Check sheet for the modelled part. Datum: model origin and axes. Units: mm. Coordinates: 2 decimals unless noted, no trailing zeros. Write each loop counter-clockwise with the first axis right and the second up, starting at its lowest first coordinate (ties: lowest second). Pieces come first, ordered by that corner, then holes. Notation, with made-up numbers: M 30,-9.75 L 81,-9.75 A12 cw 81,-4.75 Z; hole C -19.5,38.25 d6. An arc over 180 degrees is marked long. Answer as CSV lines item,"result". Start each with the question number.
1) Draft check along X on faces 1 (the cylindrical face through (-40.4, -86.24, 3.94)), 2 (the cylindrical face through (21.758, -75.637, 3.944)), 3 (the cylindrical face through (-1.788, -84.054, 3.944)), 4 (the flat face through (1, -33, 0)). Enter one of: +X half, -X half, draft (parallel to the pull), parting line (faces both ways), or undercut.
2) Material ranges on L1, parallel to X at y = -4.5, z = 4; L2, parallel to Y at x = -27, z = 1.75; L3, parallel to Y at x = -30, z = 6, recorded low to high. Write a range as [from, to].
3) Go/stop test with flat-tipped pins: pin 1 Ø21.5 at (x, y) = (30, -76) entering from -Z; pin 2 Ø4 at (y, z) = (-11.5, 6.5) entering from +X. Record where each tip stops, or that it passes through.
4) Section check C-C (x = -31.5). Record the cut outline in (y, z), and give its area (3 significant figures).
5) Section check B-B (z = 2.5). Record the cut outline in (x, y).
6) Section check A-A (y = -76). Record the cut outline in (x, z), and give its area (3 significant figures).
7) Section check D-D (x = 0). Record the cut outline in (y, z).
from build123d import *

# Parameters (mm, degrees)
SKETCH_R   = 8
SKETCH_R_2 = 8.25
PAD_DEPTH  = 8


with BuildPart() as part:
    # Sketch → Pad (new body)
    with BuildSketch(Plane.XY):
        with BuildLine():
            Line((-43.25, -79.25), (-43.25, -29.25))
            ThreePointArc((-39.101298, -16.231558), (-42.18775, -22.418244), (-43.25, -29.25))
            Line((-39.101298, -16.231558), (-18.351298, 13.018442))
            ThreePointArc((18.351298, 13.018442), (0, 22.5), (-18.351298, 13.018442))
            Line((39.101298, -16.231558), (18.351298, 13.018442))
            ThreePointArc((43.25, -29.25), (42.18775, -22.418244), (39.101298, -16.231558))
            Line((43.25, -79.25), (43.25, -29.25))
            ThreePointArc((33.25, -89.25), (40.321068, -86.321068), (43.25, -79.25))
            Line((-33.25, -89.25), (33.25, -89.25))
            ThreePointArc((-43.25, -79.25), (-40.321068, -86.321068), (-33.25, -89.25))
        make_face()
        Circle(SKETCH_R, mode=Mode.SUBTRACT)
        with Locations((0, -76)):
            Circle(SKETCH_R_2, mode=Mode.SUBTRACT)
        with Locations((30, -76)):
            Circle(SKETCH_R_2, mode=Mode.SUBTRACT)
        with Locations((-30, -76)):
            Circle(SKETCH_R_2, mode=Mode.SUBTRACT)
    extrude(amount=PAD_DEPTH)


solid = part.part
Results found:
1,face 1,"-X half"
1,face 2,"undercut"
1,face 3,"undercut"
1,face 4,"draft"
2,L1,"x = [-30.78, -6.61], [6.61, 30.78]"
2,L2,"y = [-89.25, -83.69], [-68.31, 0.83]"
2,L3,"y = [-89.25, -84.25], [-67.75, -3.4]"
3,pin 1,"stops at z = 0"
3,pin 2,"stops at x = 37.16"
4,outline,"M -89.25,0 L -84.11,0 L -84.11,8 L -89.25,8 Z; M -67.89,0 L -5.52,0 L -5.52,8 L -67.89,8 Z"
4,area,"540 mm2"
5,outline,"M -43.25,-79.25 A10 ccw -33.25,-89.25 L 33.25,-89.25 A10 ccw 43.25,-79.25 L 43.25,-29.25 A22.5 ccw 39.1,-16.23 L 18.35,13.02 A22.5 ccw -18.35,13.02 L -39.1,-16.23 A22.5 ccw -43.25,-29.25 Z; hole C -30,-76 d16.5; hole C 0,-76 d16.5; hole C 0,0 d16; hole C 30,-76 d16.5"
6,outline,"M -43.25,0 L -38.25,0 L -38.25,8 L -43.25,8 Z; M -21.75,0 L -8.25,0 L -8.25,8 L -21.75,8 Z; M 8.25,0 L 21.75,0 L 21.75,8 L 8.25,8 Z; M 38.25,0 L 43.25,0 L 43.25,8 L 38.25,8 Z"
6,area,"296 mm2"
7,outline,"M -89.25,0 L -84.25,0 L -84.25,8 L -89.25,8 Z; M -67.75,0 L -8,0 L -8,8 L -67.75,8 Z; M 8,0 L 22.5,0 L 22.5,8 L 8,8 Z"
